For this review, take the finished solid that the model builds, in its own axes (mm). Give positions to 0.01 mm unless a question says otherwise; leave off trailing zeros. Write each loop counter-clockwise with the first axis right and the second up, starting at its lowest first coordinate (ties: lowest second). Pieces come first, ordered by that corner, then holes.
1) We need section B-B on x = 735.5. Give the boundary of the cut face in (y, z), and give its area (3 significant figures).
2) We need section D-D on z = 178. Give the boundary of the cut face in (x, y).
3) For P1, Ø1, axis at y = 80, z = 152, coming from the -X side; P2, Ø3, axis at y = 117.5, z = 58.5, coming from the -X side; P3, Ø1, axis at x = 92, z = 130, coming from the +Y side, all flat-tipped, find the tip position at first contact; note any pin that passes through.
4) Wall thickness on line 1 along X through (y, z) = (179, 49); line 2 along X through (y, z) = (174.5, 90); line 3 along Y through (x, z) = (132, 163.5): over which ranges is each line inside the solid? List them lowest first.
5) We need section A-A on z = 111. Give the boundary of the cut face in (x, y).
6) We need section C-C on y = 117.5. Give the boundary of the cut face in (x, z), and give its area (3 significant figures).
Autodesk Inventor part; units mm, degrees
ref_plane "YZ Plane" through (0, 0, 0) normal (1, 0, 0) x (0, 1, 0)
ref_plane "XZ Plane" through (0, 0, 0) normal (0, 1, 0) x (-1, 0, 0)
ref_plane "XY Plane" through (0, 0, 0) normal (0, 0, 1) x (1, 0, 0)
sketch "Sketch1" plane through (0, 0, 0) normal (1, 0, 0) x (0, 1, 0)
  line L0 (0, 0) -> (190.5, 0)
  line L1 (0, 0) -> (0, 190.5)
  line L2 (0, 190.5) -> (101.6, 190.5)
  line L3 (190.5, 0) -> (190.5, 101.6)
  line L4 (190.5, 101.6) -> (101.6, 190.5)
  dimension "d0" = 190.5
  dimension "d1" = 190.5
  dimension "d2" = 101.6
  dimension "d3" = 101.6
  dimension "d4" = 88.9
  dimension "d5" = 88.9
extrude "Extrusion1" add sketch "Sketch1" along normal blind 406.4
sketch "Sketch2" plane through (0, 0, 190.5) normal (0, 0, 1) x (1, 0, 0)
  line L0 (0, 0) -> (0, 190.5)
  line L1 (0, 190.5) -> (88.9, 190.5)
  line L2 (0, 190.5) -> (406.4, 190.5)
  line L3 (0, 190.5) -> (0, 101.6)
  line L4 (0, 101.6) -> (88.9, 190.5)
  dimension "d8" = 88.9
  dimension "d9" = 88.9
extrude "Extrusion2" cut sketch "Sketch2" against normal up to surface (190.5 mm away)
mirror "Mirror1" about plane through (406.4, 95.25, 95.25) normal (1, 0, 0) of "Extrusion1", "Extrusion2"
properties part number "Return_L" material "Limestone"
Results list:
1. outline: (0, 0) - (178.9, 0) - (178.9, 113.2) - (101.6, 190.5) - (0, 190.5) - close
1. area: 31,100 mm2
2. outline: (0, 0) - (812.8, 0) - (812.8, 101.6) - (800.3, 114.1) - (12.5, 114.1) - (0, 101.6) - close
3. P1: stops at x = 0
3. P2: stops at x = 14.4
3. P3: stops at y = 162.6
4. line 1: x = 77.4 to 735.4
4. line 2: x = 72.9 to 739.9
4. line 3: y = 0 to 128.6
5. outline: (0, 0) - (812.8, 0) - (812.8, 101.6) - (733.3, 181.1) - (79.5, 181.1) - (0, 101.6) - close
6. outline: (15.9, 0) - (796.9, 0) - (796.9, 174.6) - (15.9, 174.6) - close
6. area: 136,000 mm2
